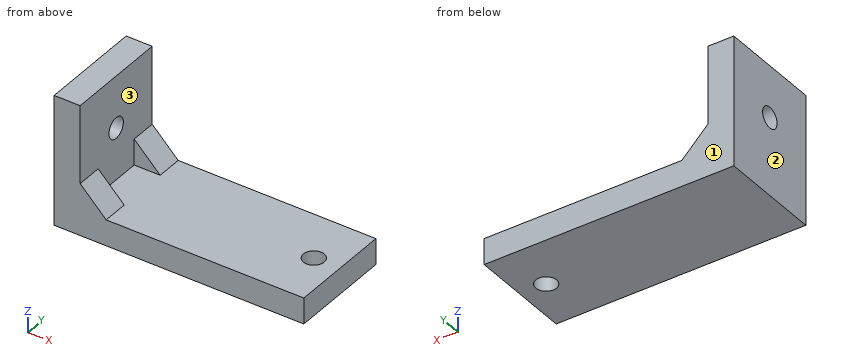
from build123d import *

# Parameters (mm, degrees)
SKETCH1_W           = 48
SKETCH1_H           = 20
BOSS_EXTRUDE1_DEPTH = 5
SKETCH2_W           = 5
SKETCH2_H           = 20
BOSS_EXTRUDE2_DEPTH = 20
SKETCH3_R           = 2
CUT_EXTRUDE1_DEPTH  = 51.734603576
SKETCH5_W           = 5
SKETCH5_H           = 5
BOSS_EXTRUDE3_DEPTH = 5
CUT_EXTRUDE3_DEPTH  = 41.012498047
SKETCH7_R           = 2
CUT_EXTRUDE4_DEPTH  = 37.069377594


with BuildPart() as part:
    # Sketch1 → Boss-Extrude1 (new body)
    with BuildSketch(Plane.XY):
        Rectangle(SKETCH1_W, SKETCH1_H)
    extrude(amount=BOSS_EXTRUDE1_DEPTH)

    # Sketch2 → Boss-Extrude2 (add)
    with BuildSketch(Plane.XY.offset(5)):
        with Locations((-21.5, 0)):
            Rectangle(SKETCH2_W, SKETCH2_H)
    extrude(amount=BOSS_EXTRUDE2_DEPTH)

    # Sketch3 → Cut-Extrude1 (cut, through all)
    with BuildSketch(Plane(origin=(-19, 0, 0), x_dir=(0, 0, -1), z_dir=(1, 0, 0))):
        with Locations((-15, 0)):
            Circle(SKETCH3_R)
    extrude(amount=-CUT_EXTRUDE1_DEPTH, mode=Mode.SUBTRACT)

    # Sketch5 → Boss-Extrude3 (add)
    with BuildSketch(Plane(origin=(-19, 0, 0), x_dir=(0, 0, -1), z_dir=(1, 0, 0))):
        with Locations((-7.5, -7.5)):
            Rectangle(SKETCH5_W, SKETCH5_H)
        with Locations((-7.5, 7.5)):
            Rectangle(SKETCH5_W, SKETCH5_H)
    extrude(amount=BOSS_EXTRUDE3_DEPTH)

    # Sketch6 → Cut-Extrude3 (cut, through all)
    with BuildSketch(Plane(origin=(0, 10, 0), x_dir=(1, 0, 0), z_dir=(0, 1, 0))):
        Polygon((-14, -5), (-19, -10), (-14, -10), align=None)
    extrude(amount=-CUT_EXTRUDE3_DEPTH, mode=Mode.SUBTRACT)

    # Sketch7 → Cut-Extrude4 (cut, through all)
    with BuildSketch(Plane(origin=(0, 0, 0), x_dir=(-1, 0, 0), z_dir=(0, 0, -1))):
        with Locations((-19, 0)):
            Circle(SKETCH7_R)
    extrude(amount=-CUT_EXTRUDE4_DEPTH, mode=Mode.SUBTRACT)


solid = part.part
CAD build for the part. Positions are in the model's coordinates, mm. Face numbers are marked on the shaded views. Coordinates: 2 decimals unless noted, no trailing zeros. Loops run counter-clockwise (first coordinate to the right, second up) from the corner with the lowest first, then second, coordinate; pieces in that order, holes last. Notation, with made-up numbers: (37.5, 24) - (65.5, 24) arc R12 cw to (65.5, 41) - close; hole circle Ø5 at (7.25, 67.5). An arc over 180 degrees is marked (long way). Use one line per item in the form item = value. Start each with the question number.
1) Flat gauge pins, fed straight in: pin 1 (10 mm diameter, centred on x = -18, y = -5.5, fed in from -Z); pin 2 (12 mm diameter, centred on x = -10.5, z = 18.5, fed in from +Y); pin 3 (3 mm diameter, centred on x = -4, y = -0.5, fed in from +Z); pin 4 (4 mm diameter, centred on x = -16, y = -6, fed in from +Z). Where does each tip first touch, or does it go through?
2) Band-saw the part on C-C (y = 0). Give the cut face in (x, z), and give its area (3 significant figures).
3) Two-plate mould, pull along Y, no slides. Class the marked faces 1, 2 and 3: +Y half, -Y half, draft (parallel to the pull), parting line (faces both ways), or undercut.
4) Drill centre lines: L1, parallel to Y at x = -20.65, z = 15; L2, parallel to Z at x = 0.5, y = -1; L3, parallel to X at y = 0.5, z = 8. Where is each one in solid material? Low to high. Write a range as from..to.
5) Band-saw the part on D-D (x = -20). Give the cut face in (y, z).
6) Band-saw the part on B-B (x = 19). Give the cut face in (y, z).
7) Band-saw the part on A-A (z = 15). Give the cut face in (x, y), and give its area (3 significant figures).
Check values:
q1.pin_1 = 0
q1.pin_2 = through
q1.pin_3 = 5
q1.pin_4 = 9
q2.outline = (-24, 0) - (17, 0) - (17, 5) - (-19, 5) - (-19, 13) - (-24, 13) - close; (-24, 17) - (-19, 17) - (-19, 25) - (-24, 25) - close; (21, 0) - (24, 0) - (24, 5) - (21, 5) - close
q2.area = 300 mm2
q3.face_1 = +Y half
q3.face_2 = draft
q3.face_3 = undercut
q4.L1 = -10..-2, 2..10
q4.L2 = 0..5
q4.L3 = -24..-19
q5.outline = (-10, 0) - (10, 0) - (10, 25) - (-10, 25) - close; hole circle Ø4 at (0, 15)
q6.outline = (-10, 0) - (-2, 0) - (-2, 5) - (-10, 5) - close; (2, 0) - (10, 0) - (10, 5) - (2, 5) - close
q7.outline = (-24, -10) - (-19, -10) - (-19, -2) - (-24, -2) - close; (-24, 2) - (-19, 2) - (-19, 10) - (-24, 10) - close
q7.area = 80.0 mm2
